The listing builds one solid part. Answer for the finished solid, in the listing's coordinates (mm). A direction names the side the tool comes from. Coordinates: 2 decimals unless noted, no trailing zeros. Loops run counter-clockwise (first coordinate to the right, second up) from the corner with the lowest first, then second, coordinate; pieces in that order, holes last. Notation, with made-up numbers: M -20.5,6 L 8.5,6 A27 cw 8.5,42 Z; hole C 41.25,-22.5 d4. An arc over 180 degrees is marked long. Answer in a Markdown table with one row per item. Add a question column.
from build123d import *

# Parameters (mm, degrees)
BOSS_EXTRUDE1_DEPTH      = 15
BOSS_EXTRUDE1_DEPTH_BACK = 10
SKETCH3_R                = 1.5
CUT_EXTRUDE2_DEPTH       = 9


with BuildPart() as part:
    # Sketch2 → Boss-Extrude1 (new body, two sides)
    with BuildSketch(Plane(origin=(0, 0, 0), x_dir=(0, 0, -1), z_dir=(1, 0, 0))) as boss_extrude1_sk:
        Polygon((-10, 8), (-10, 308), (10, 308), (10, 8), (31, 8), (31, 0), (-29, 0), (-29, 8), align=None)
    extrude(amount=BOSS_EXTRUDE1_DEPTH)
    extrude(boss_extrude1_sk.sketch, amount=-BOSS_EXTRUDE1_DEPTH_BACK)

    # Sketch3 → Cut-Extrude2 (cut, through all)
    with BuildSketch(Plane(origin=(0, 8, 0), x_dir=(1, 0, 0), z_dir=(0, 1, 0))):
        with Locations((1.863320083, -22)):
            Circle(SKETCH3_R)
    cut_extrude2 = extrude(amount=-CUT_EXTRUDE2_DEPTH, mode=Mode.SUBTRACT)

    # Mirror2: Cut-Extrude2 across plane
    add(cut_extrude2.mirror(Plane.XY), mode=Mode.SUBTRACT)


solid = part.part
(1) A cutting plane is placed at A-A (x = -6.5). Give the vertices of the cut face in (y, z), plus the area to 3 significant figures.
(2) Each of these flat-tipped pins is pushed along its axis until it touches: pin 1 (12 mm diameter, centred on x = 9, z = -23.5, fed in from +Y); pin 2 (5 mm diameter, centred on x = 0.5, y = 235.5, fed in from -Z). Where does it stop, or does it pass through?
(3) Straight lines are drawn through the part: line 1 (X direction, y = 5, z = 22); line 2 (Z direction, x = 5.5, y = 130); line 3 (Y direction, x = 3.25, z = -28). For each, find the intervals that lie inside material, in ascending order.
(4) For faces 1 (the face through (3, 8, 20)), 2 (the face through (3, 0, -1)), 3 (the face through (3, 8, -20)), determine the directions among +Z, -Z, +X, -X, +Y, -Y from which every point of the face is accessible in a straight line to the end or side of a thin tool.
(5) A cutting plane is placed at B-B (y = 99.5). Give the vertices of the cut face in (x, z).
Solved:
| question | item | result |
|---|---|---|
| 1 | outline | M 0,-31 L 8,-31 L 8,-10 L 308,-10 L 308,10 L 8,10 L 8,29 L 0,29 Z |
| 1 | area | 6,480 mm² |
| 2 | pin 1 | stops at y = 8 |
| 2 | pin 2 | stops at z = -10 |
| 3 | line 1 | x = -10 to 0.36, 3.36 to 15 |
| 3 | line 2 | z = -10 to 10 |
| 3 | line 3 | y = 0 to 8 |
| 4 | face 1 | +Z, +X, -X, +Y |
| 4 | face 2 | +Z, -Z, +X, -X, -Y |
| 4 | face 3 | -Z, +X, -X, +Y |
| 5 | outline | M -10,-10 L 15,-10 L 15,10 L -10,10 Z |
